Model file for the job. Use its own axes, mm. Face numbers are marked on the shaded views. Give positions to 0.01 mm unless a question says otherwise; leave off trailing zeros. Loops run counter-clockwise (first coordinate to the right, second up) from the corner with the lowest first, then second, coordinate; pieces in that order, holes last. Notation, with made-up numbers: (9, 62) - (62, 62) arc R14 ccw to (62, 75) - close; hole circle Ø9 at (-7.5, -18). An arc over 180 degrees is marked (long way). Use a Markdown table: item, result.
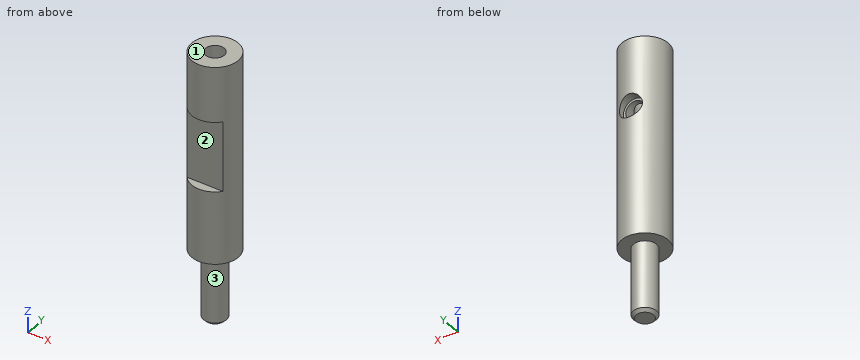
Autodesk Inventor part; units mm, degrees
ref_plane "Work Plane1" through (0, 4, 34) normal (0, 1, 0) x (-1, 0, 0)
ref_plane "Work Plane2" through (0, 0, 0) normal (1, 0, 0) x (0, 1, 0)
ref_plane "Work Plane3" through (0, 4, 0) normal (0, 1, 0) x (-1, 0, 0)
sketch "Sketch1" plane through (0, 0, 0) normal (0, 0, 1) x (1, 0, 0)
  circle A0 centre (0, 0) radius 4
  dimension "d0" = 8
extrude "Extrusion1" add sketch "Sketch1" along normal blind 34
sketch "Sketch2" plane through (0, 0, 0) normal (0, 0, -1) x (-1, 0, 0)
  circle A0 centre (0, 0) radius 2
  dimension "d3" = 4
extrude "Extrusion2" add sketch "Sketch2" along normal blind 12
chamfer "Chamfer1" distance 0.5 angle 45 1 edges at (2, 0, -12)
sketch "Sketch3" plane through (0, 0, 34) normal (0, 0, 1) x (1, 0, 0)
  line L0 (0, 0) -> (0, 4)
  circle A0 centre (0, 0) radius 4
hole "Hole1" at (0, 0, 34) direction (0, 0, -1) diameter 3.2 depth 14 tip angle 118
ref_plane "Work Plane1" through (0, 4, 34) normal (0, 1, 0) x (-1, 0, 0)
ref_plane "Work Plane2" through (0, 0, 0) normal (1, 0, 0) x (0, 1, 0)
sketch "Sketch5" plane through (0, 0, 0) normal (1, 0, 0) x (0, 1, 0)
  line L0 (-4, 0) -> (-4, 34)
  line L1 (-4, 24.5) -> (-2.5, 24.5)
  line L2 (-2.5, 24.5) -> (-2.5, 12.5)
  line L3 (-2.5, 12.5) -> (-4, 12.5)
  line L4 (-4, 12.5) -> (-4, 24.5)
  line L5 (4, 34) -> (-4, 34)
  point P0 (0, 0)
  dimension "d19" = 12
  dimension "d20" = 9.5
  dimension "d21" = 1.5
extrude "Extrusion3" cut sketch "Sketch5" along normal mid plane 100
ref_plane "Work Plane3" through (0, 4, 0) normal (0, 1, 0) x (-1, 0, 0)
sketch "Sketch6" plane through (0, 4, 0) normal (0, 1, 0) x (-1, 0, 0)
  line L0 (4, 34) -> (-4, 34)
  line L1 (0, 34) -> (0, 22.5)
  point P0 (0, 0)
  dimension "d25" = 11.5
hole "Hole2" at (0, 4, 22.5) direction (0, -1, 0) diameter 4 depth 1.5
hole "Hole3" at (0, 4, 22.5) direction (0, -1, 0) diameter 3.2 depth 4 tip angle 118
properties part number "KURBELWELLE PART 7" material "Stainless Steel"
(1) Drill centre lines: probe 1 along Y at (x, z) = (0, 25); probe 2 along X at (y, z) = (2.5, 10.5); probe 3 along Z at (x, y) = (-2.5, 0). Where is each one in solid material? Low to high. Write a range as [from, to].
Computed:
| item | result |
|---|---|
| probe 1 | [-4, -1.6], [1.6, 4] |
| probe 2 | [-3.12, 3.12] |
| probe 3 | [0, 34] |
(2) Slice it at A-A, the plane y = -3.5. Write the cut outline in (x, z), plus the area to 3 significant figures.
Computed:
| item | result |
|---|---|
| outline | (-1.94, 0) - (1.94, 0) - (1.94, 12.5) - (-1.94, 12.5) - close; (-1.94, 24.5) - (1.94, 24.5) - (1.94, 34) - (-1.94, 34) - close |
| area | 85.2 mm² |
(3) Pin check, flat tips, straight feed: P1, Ø2.5, axis at x = 0, z = 22.5, coming from the -Y side; P2, Ø3, axis at y = -3, z = 25.5, coming from the -X side; P3, Ø1.2, axis at x = 0.5, z = 22.5, coming from the +Y side. Stop position of each tip, or through.
Computed:
| item | result |
|---|---|
| P1 | y = -2.5 |
| P2 | x = -3.71 |
| P3 | y = -1.16 |
(4) Slice it at D-D, the plane z = 22.5. Write the cut outline in (x, y), plus the area to 3 significant figures.
Computed:
| item | result |
|---|---|
| outline | (-3.12, -2.5) - (3.12, -2.5) arc R4 ccw to (2, 3.46) - (2, 2.5) - (1.6, 2.5) - (1.6, 0) arc R1.6 cw to (-1.6, 0) - (-1.6, 2.5) - (-2, 2.5) - (-2, 3.46) arc R4 ccw to start |
| area | 26.4 mm² |
(5) Slice it at C-C, the plane z = 27.5. Write the cut outline in (x, y), plus the area to 3 significant figures.
Computed:
| item | result |
|---|---|
| outline | circle Ø8 at (0, 0); hole circle Ø3.2 at (0, 0) |
| area | 42.2 mm² |
(6) Slice it at B-B, the plane x = -2.5. Write the cut outline in (y, z), plus the area to 3 significant figures.
Computed:
| item | result |
|---|---|
| outline | (-3.12, 0) - (3.12, 0) - (3.12, 34) - (-3.12, 34) - (-3.12, 24.5) - (-2.5, 24.5) - (-2.5, 12.5) - (-3.12, 12.5) - close |
| area | 205 mm² |
(7) Mould opens along Z. For the marked faces 1, 2 and 3 say: pulls with the +Z half, pulls with the -Z half, needs draft (parallel to the pull), parting line crosses it, or undercut.
Computed:
| item | result |
|---|---|
| face 1 | pulls with the +Z half |
| face 2 | undercut |
| face 3 | needs draft |
